```python
from build123d import *

# Parameters (mm, degrees)
SKETCH_1_R          = 1.6
SKETCH_1_W          = 15.2
SKETCH_1_H          = 15.2
EXTRUDE_1_DEPTH     = 19.5
CUT_EXTRUDE_1_DEPTH = 14.5
SKETCH_3_W          = 23.2
SKETCH_3_H          = 23.2
SKETCH_3_W_2        = 15.2
SKETCH_3_H_2        = 15.2
EXTRUDE_2_DEPTH     = 20
FILLET_1_R          = 4
FILLET_2_R          = 6
CHAMFER_1_SIZE      = 1.5
CHAMFER_2_SIZE      = 1
SKETCH_4_R          = 1.6
CUT_EXTRUDE_2_DEPTH = 68.026114314
SKETCH_5_R          = 1.6
CUT_EXTRUDE_3_DEPTH = 68.026114314
FILLET_3_R          = 5


with BuildPart() as part:
    # 草图1 → 凸台-拉伸1 (new body)
    with BuildSketch(Plane(origin=(0, 0, 0), x_dir=(0, 0, -1), z_dir=(1, 0, 0))):
        Polygon((12.5, -30.7), (30.7, -30.7), (30.7, -12.5), (40, -12.5), (40, 12.5), (-12.5, 12.5), (-12.5, -40), (12.5, -40), align=None)
        with Locations((10, 0)):
            Circle(SKETCH_1_R, mode=Mode.SUBTRACT)
        with Locations((30, 0)):
            Circle(SKETCH_1_R, mode=Mode.SUBTRACT)
        with Locations(Location((0, -30, 0), (0, 0, 180))):
            Circle(SKETCH_1_R, mode=Mode.SUBTRACT)
        with Locations(Location((0, -10, 0), (0, 0, 180))):
            Circle(SKETCH_1_R, mode=Mode.SUBTRACT)
        with Locations((15.1, -15.1)):
            Rectangle(SKETCH_1_W, SKETCH_1_H, mode=Mode.SUBTRACT)
    extrude(amount=EXTRUDE_1_DEPTH)

    # 草图2 → 切除-拉伸1 (cut)
    with BuildSketch(Plane.ZY):
        Polygon((7.5, 7.5), (7.5, -40), (-7.5, -40), (-7.5, -7.5), (-40, -7.5), (-40, 7.5), align=None)
    extrude(amount=-CUT_EXTRUDE_1_DEPTH, mode=Mode.SUBTRACT)

    # 草图3 → 凸台-拉伸2 (add)
    with BuildSketch(Plane(origin=(19.5, 0, 0), x_dir=(0, 0, -1), z_dir=(1, 0, 0))):
        with Locations((15.1, -15.1)):
            Rectangle(SKETCH_3_W, SKETCH_3_H)
        with Locations((15.1, -15.1)):
            Rectangle(SKETCH_3_W_2, SKETCH_3_H_2, mode=Mode.SUBTRACT)
    extrude(amount=EXTRUDE_2_DEPTH)

    # 圆角1
    # the kernel refuses this fillet: 4 mm, written as the material it adds along each edge
    with BuildSketch(Plane(origin=(19.5, -3.5, -3.5), x_dir=(0, 0, 1), z_dir=(0, -1, 0))) as fillet_1_piece_1_section:
        with BuildLine():
            CenterArc((FILLET_1_R, -FILLET_1_R), FILLET_1_R, 90, 90)
            Line((0, -FILLET_1_R), (0, 0))
            Line((0, 0), (FILLET_1_R, 0))
        make_face()
    fillet_1_piece_1 = extrude(amount=23.2, mode=Mode.PRIVATE)
    fillet_1_piece_1 = fillet_1_piece_1 - Plane(origin=(20.41689995, -10, 0), x_dir=(0, 0, 1), z_dir=(-1, 0, 0)) * Cylinder(1.6, 63, mode=Mode.PRIVATE)
    add(fillet_1_piece_1)
    with BuildSketch(Plane(origin=(19.5, -26.7, -3.5), x_dir=(0, -1, 0), z_dir=(0, 0, -1)), Plane(origin=(19.5, -26.7, -26.7), x_dir=(0, 0, -1), z_dir=(0, 1, 0))) as fillet_1_piece_2:
        with BuildLine():
            CenterArc((FILLET_1_R, -FILLET_1_R), FILLET_1_R, 90, 90)
            Line((0, -FILLET_1_R), (0, 0))
            Line((0, 0), (FILLET_1_R, 0))
        make_face()
    extrude(amount=23.2)
    with BuildSketch(Plane(origin=(19.5, -3.5, -26.7), x_dir=(0, 1, 0), z_dir=(0, 0, 1))) as fillet_1_piece_3_section:
        with BuildLine():
            CenterArc((FILLET_1_R, -FILLET_1_R), FILLET_1_R, 90, 90)
            Line((0, -FILLET_1_R), (0, 0))
            Line((0, 0), (FILLET_1_R, 0))
        make_face()
    fillet_1_piece_3 = extrude(amount=23.2, mode=Mode.PRIVATE)
    fillet_1_piece_3 = fillet_1_piece_3 - Plane(origin=(20.416900014, 0, -10), x_dir=(0, 0, -1), z_dir=(-1, 0, 0)) * Cylinder(1.6, 63, mode=Mode.PRIVATE)
    add(fillet_1_piece_3)
    with BuildSketch(Plane(origin=(19.5, -3.5, -26.7), x_dir=(0, 1, 0), z_dir=(0, 0, 1))) as fillet_1_piece_4a_section:
        with BuildLine():
            CenterArc((FILLET_1_R, -FILLET_1_R), FILLET_1_R, 90, 90)
            Line((0, -FILLET_1_R), (0, 0))
            Line((0, 0), (FILLET_1_R, 0))
        make_face()
    fillet_1_piece_4a = extrude(amount=33.2, mode=Mode.PRIVATE)
    fillet_1_piece_4a = split(fillet_1_piece_4a, bisect_by=Plane(origin=(20.405580457, -2.594419543, -3.5), z_dir=(0, 0, 1)), keep=Keep.TOP, mode=Mode.PRIVATE)
    with BuildSketch(Plane(origin=(19.5, 6.5, -3.5), x_dir=(0, 0, 1), z_dir=(0, -1, 0))) as fillet_1_piece_4b_section:
        with BuildLine():
            CenterArc((FILLET_1_R, -FILLET_1_R), FILLET_1_R, 90, 90)
            Line((0, -FILLET_1_R), (0, 0))
            Line((0, 0), (FILLET_1_R, 0))
        make_face()
    fillet_1_piece_4b = extrude(amount=33.2, mode=Mode.PRIVATE)
    fillet_1_piece_4b = split(fillet_1_piece_4b, bisect_by=Plane(origin=(20.405580457, -3.5, -2.594419543), z_dir=(0, 1, 0)), keep=Keep.TOP, mode=Mode.PRIVATE)
    fillet_1_piece_4 = fillet_1_piece_4a & fillet_1_piece_4b
    add(fillet_1_piece_4)
    with BuildSketch(Plane(origin=(19.5, -26.7, 6.5), x_dir=(0, -1, 0), z_dir=(0, 0, -1))) as fillet_1_piece_5a_section:
        with BuildLine():
            CenterArc((FILLET_1_R, -FILLET_1_R), FILLET_1_R, 90, 90)
            Line((0, -FILLET_1_R), (0, 0))
            Line((0, 0), (FILLET_1_R, 0))
        make_face()
    fillet_1_piece_5a = extrude(amount=33.2, mode=Mode.PRIVATE)
    fillet_1_piece_5a = fillet_1_piece_5a - Plane(origin=(20.438690709, -30, 0), x_dir=(0, 0, 1), z_dir=(-1, 0, 0)) * Cylinder(1.6, 83, mode=Mode.PRIVATE)
    fillet_1_piece_5a = split(fillet_1_piece_5a, bisect_by=Plane(origin=(20.438690709, -27.535460333, -3.5), z_dir=(0, 0, 1)), keep=Keep.TOP, mode=Mode.PRIVATE)
    with BuildSketch(Plane(origin=(19.5, -3.5, -3.5), x_dir=(0, 0, 1), z_dir=(0, -1, 0))) as fillet_1_piece_5b_section:
        with BuildLine():
            CenterArc((FILLET_1_R, -FILLET_1_R), FILLET_1_R, 90, 90)
            Line((0, -FILLET_1_R), (0, 0))
            Line((0, 0), (FILLET_1_R, 0))
        make_face()
    fillet_1_piece_5b = extrude(amount=33.2, mode=Mode.PRIVATE)
    fillet_1_piece_5b = fillet_1_piece_5b - Plane(origin=(20.432327139, -30, 0), x_dir=(0, 0, 1), z_dir=(-1, 0, 0)) * Cylinder(1.6, 83, mode=Mode.PRIVATE)
    fillet_1_piece_5b = split(fillet_1_piece_5b, bisect_by=Plane(origin=(20.432327139, -26.7, -2.653974982), z_dir=(0, -1, 0)), keep=Keep.TOP, mode=Mode.PRIVATE)
    fillet_1_piece_5 = fillet_1_piece_5a & fillet_1_piece_5b
    add(fillet_1_piece_5)
    with BuildSketch(Plane(origin=(19.5, -26.7, -3.5), x_dir=(0, -1, 0), z_dir=(0, 0, -1))) as fillet_1_piece_6a_section:
        with BuildLine():
            CenterArc((FILLET_1_R, -FILLET_1_R), FILLET_1_R, 90, 90)
            Line((0, -FILLET_1_R), (0, 0))
            Line((0, 0), (FILLET_1_R, 0))
        make_face()
    fillet_1_piece_6a = extrude(amount=33.2, mode=Mode.PRIVATE)
    fillet_1_piece_6a = split(fillet_1_piece_6a, bisect_by=Plane(origin=(20.405580457, -27.605580457, -30.7), z_dir=(0, 0, 1)), keep=Keep.TOP, mode=Mode.PRIVATE)
    fillet_1_piece_6a = split(fillet_1_piece_6a, bisect_by=Plane(origin=(20.405580457, -27.605580457, -26.7), z_dir=(0, 0, -1)), keep=Keep.TOP, mode=Mode.PRIVATE)
    with BuildSketch(Plane(origin=(19.5, -36.7, -26.7), x_dir=(0, 0, -1), z_dir=(0, 1, 0))) as fillet_1_piece_6b_section:
        with BuildLine():
            CenterArc((FILLET_1_R, -FILLET_1_R), FILLET_1_R, 90, 90)
            Line((0, -FILLET_1_R), (0, 0))
            Line((0, 0), (FILLET_1_R, 0))
        make_face()
    fillet_1_piece_6b = extrude(amount=33.2, mode=Mode.PRIVATE)
    fillet_1_piece_6b = split(fillet_1_piece_6b, bisect_by=Plane(origin=(20.405580457, -30.7, -27.605580457), z_dir=(0, 1, 0)), keep=Keep.TOP, mode=Mode.PRIVATE)
    fillet_1_piece_6b = split(fillet_1_piece_6b, bisect_by=Plane(origin=(20.405580457, -26.7, -27.605580457), z_dir=(0, -1, 0)), keep=Keep.TOP, mode=Mode.PRIVATE)
    fillet_1_piece_6 = fillet_1_piece_6a & fillet_1_piece_6b
    add(fillet_1_piece_6)
    with BuildSketch(Plane(origin=(19.5, -26.7, -26.7), x_dir=(0, 0, -1), z_dir=(0, 1, 0))) as fillet_1_piece_7a_section:
        with BuildLine():
            CenterArc((FILLET_1_R, -FILLET_1_R), FILLET_1_R, 90, 90)
            Line((0, -FILLET_1_R), (0, 0))
            Line((0, 0), (FILLET_1_R, 0))
        make_face()
    fillet_1_piece_7a = extrude(amount=33.2, mode=Mode.PRIVATE)
    fillet_1_piece_7a = fillet_1_piece_7a - Plane(origin=(20.438690575, 0, -30), x_dir=(0, 0, -1), z_dir=(-1, 0, 0)) * Cylinder(1.6, 83, mode=Mode.PRIVATE)
    fillet_1_piece_7a = split(fillet_1_piece_7a, bisect_by=Plane(origin=(20.438690575, -3.5, -27.535460712), z_dir=(0, 1, 0)), keep=Keep.TOP, mode=Mode.PRIVATE)
    with BuildSketch(Plane(origin=(19.5, -3.5, -36.7), x_dir=(0, 1, 0), z_dir=(0, 0, 1))) as fillet_1_piece_7b_section:
        with BuildLine():
            CenterArc((FILLET_1_R, -FILLET_1_R), FILLET_1_R, 90, 90)
            Line((0, -FILLET_1_R), (0, 0))
            Line((0, 0), (FILLET_1_R, 0))
        make_face()
    fillet_1_piece_7b = extrude(amount=33.2, mode=Mode.PRIVATE)
    fillet_1_piece_7b = fillet_1_piece_7b - Plane(origin=(20.432327238, 0, -30), x_dir=(0, 0, -1), z_dir=(-1, 0, 0)) * Cylinder(1.6, 83, mode=Mode.PRIVATE)
    fillet_1_piece_7b = split(fillet_1_piece_7b, bisect_by=Plane(origin=(20.432327238, -2.653975394, -26.7), z_dir=(0, 0, -1)), keep=Keep.TOP, mode=Mode.PRIVATE)
    fillet_1_piece_7 = fillet_1_piece_7a & fillet_1_piece_7b
    add(fillet_1_piece_7)

    # 圆角2
    # the kernel refuses this fillet: 6 mm, written as the material it adds along each edge
    with BuildSketch(Plane(origin=(0, -30.7, -12.5), x_dir=(0, 0, -1), z_dir=(1, 0, 0)), Plane(origin=(0, -12.5, -30.7), x_dir=(0, 0, -1), z_dir=(1, 0, 0))) as fillet_2_piece_1:
        with BuildLine():
            CenterArc((FILLET_2_R, -FILLET_2_R), FILLET_2_R, 90, 90)
            Line((0, -FILLET_2_R), (0, 0))
            Line((0, 0), (FILLET_2_R, 0))
        make_face()
    extrude(amount=19.5)
    # the kernel refuses this fillet: 6 mm, written as the material it takes off along each edge
    with BuildSketch(Plane(origin=(-15, -30.7, -30.7), x_dir=(0, 0, 1), z_dir=(1, 0, 0))) as fillet_2_2_piece_1:
        with BuildLine():
            CenterArc((FILLET_2_R, -FILLET_2_R), FILLET_2_R, 90, 90)
            Line((0, -FILLET_2_R), (0, 0))
            Line((0, 0), (FILLET_2_R, 0))
        make_face()
    extrude(amount=49.5, mode=Mode.SUBTRACT)

    # 倒角1
    chamfer_1_edges = [part.edges().sort_by_distance(p)[0] for p in [
        (39.5, -15.1, -7.5),
        (39.5, -22.7, -15.1),
        (39.5, -15.1, -22.7),
        (39.5, -7.5, -15.1),
    ]]
    chamfer(chamfer_1_edges, length=CHAMFER_1_SIZE)

    # 倒角2
    chamfer_2_edges = [part.edges().sort_by_distance(p)[0] for p in [
        (0, 7.5, -16.25),
        (0, -7.5, -31.35),
        (0, -31.35, -7.5),
        (0, -16.25, 7.5),
    ]]
    chamfer(chamfer_2_edges, length=CHAMFER_2_SIZE)

    # 草图4 → 切除-拉伸2 (cut, through all)
    with BuildSketch(Plane.XY.offset(-3.5)):
        with Locations((32, -15.1)):
            Circle(SKETCH_4_R)
    extrude(amount=-CUT_EXTRUDE_2_DEPTH, mode=Mode.SUBTRACT)

    # 草图5 → 切除-拉伸3 (cut, through all)
    with BuildSketch(Plane(origin=(0, -3.5, 0), x_dir=(1, 0, 0), z_dir=(0, 1, 0))):
        with Locations(Location((32, 15.1, 0), (0, 0, 270))):
            Circle(SKETCH_5_R)
    extrude(amount=-CUT_EXTRUDE_3_DEPTH, mode=Mode.SUBTRACT)

    # 圆角3
    fillet_3_edges = [part.edges().sort_by_distance(p)[0] for p in [
        (9.75, 12.5, 12.5),
    ]]
    fillet(fillet_3_edges, radius=FILLET_3_R)


solid = part.part
```
Geometry check sheet. Reference: the model listing, model coordinates, mm. A direction names the side the tool comes from. Coordinates: 2 decimals unless noted, no trailing zeros. Write each loop counter-clockwise with the first axis right and the second up, starting at its lowest first coordinate (ties: lowest second). Pieces come first, ordered by that corner, then holes. Notation, with made-up numbers: (12, 25) -> (70, 25) arc R18 cw to (70, 46) -> close; hole circle Ø5 at (68, 33). An arc over 180 degrees is marked (long way). Use CSV: the item, a comma, the result in double quotes. Start each with the question number.
Item 1: Cross-section at B-B, the plane y = -10. Record the cut outline in (x, z).
Item 2: Mould release check, pull along X, two halves, no side actions. Record for faces 4 (the flat face through (30, -3.5, -15)), 5 (the cylindrical face through (31.39, -24.67, -13.62)), 6 (the flat face through (14.5, -5, -11)), 7 (the cylindrical face through (20.641, -27.903, -14.891)): released by +X, released by -X, zero draft, split by the parting line, or undercut.
Item 3: Cross-section at A-A, the plane x = 32. Record the cut outline in (y, z), plus the area to 3 significant figures.
Item 4: Cross-section at D-D, the plane x = 7. Record the cut outline in (y, z), plus the area to 3 significant figures.
Item 5: Set-up check for faces 1 (the flat face through (8, 7.5, -17)), 2 (the flat face through (38.8, -15.2, -23.5)), 3 (the flat face through (10, -30.7, -22)): record each of +Z, -Z, +X, -X, +Y, -Y from which the full face is reachable in a straight line by a thin tool's end or side.
Item 6: Depth check by flat-ended pin: pin 1 Ø17.5 at (x, z) = (32.5, -17.5) entering from +Y; pin 2 Ø2 at (x, z) = (32, -27) entering from -Y; pin 3 Ø3 at (y, z) = (2, -10.5) entering from -X; pin 4 Ø2.5 at (x, y) = (32, -15.1) entering from -Z. Enter the tip coordinate at first touch or a pass-through.
Item 7: Thickness scan on line 1 (Z direction, x = 15, y = -10); line 2 (Y direction, x = 15, z = 0). Record the ranges inside material, lowest first.
Answers:
1,outline,"(0, -40) -> (19.5, -40) -> (19.5, -30.7) arc R4 cw to (23.5, -26.7) -> (39.5, -26.7) -> (39.5, -24.2) -> (38, -22.7) -> (0, -22.7) -> close; (0, 8.5) -> (1, 7.5) -> (14.5, 7.5) -> (14.5, 1.6) -> (19.5, 1.6) -> (19.5, 12.5) -> (0, 12.5) -> close; (14.5, -7.5) -> (38, -7.5) -> (39.5, -6) -> (39.5, -3.5) -> (23.5, -3.5) arc R4 cw to (20.1, -1.6) -> (14.5, -1.6) -> close"
2,face 4,"zero draft"
2,face 5,"undercut"
2,face 6,"released by -X"
2,face 7,"released by +X"
3,outline,"(-26.7, -26.7) -> (-16.7, -26.7) -> (-16.7, -22.7) -> (-22.7, -22.7) -> (-22.7, -16.7) -> (-26.7, -16.7) -> close; (-26.7, -13.5) -> (-22.7, -13.5) -> (-22.7, -7.5) -> (-16.7, -7.5) -> (-16.7, -3.5) -> (-26.7, -3.5) -> close; (-13.5, -26.7) -> (-3.5, -26.7) -> (-3.5, -16.7) -> (-7.5, -16.7) -> (-7.5, -22.7) -> (-13.5, -22.7) -> close; (-13.5, -7.5) -> (-7.5, -7.5) -> (-7.5, -13.5) -> (-3.5, -13.5) -> (-3.5, -3.5) -> (-13.5, -3.5) -> close"
3,area,"256 mm^2"
4,outline,"(-40, -12.5) -> (-36.7, -12.5) arc R6 cw to (-30.7, -18.5) -> (-30.7, -24.7) arc R6 ccw to (-24.7, -30.7) -> (-18.5, -30.7) arc R6 cw to (-12.5, -36.7) -> (-12.5, -40) -> (-7.5, -40) -> (-7.5, -22.7) -> (-22.7, -22.7) -> (-22.7, -7.5) -> (-40, -7.5) -> close; (-40, 7.5) -> (7.5, 7.5) -> (7.5, -40) -> (12.5, -40) -> (12.5, 7.5) arc R5 ccw to (7.5, 12.5) -> (-40, 12.5) -> close"
4,area,"903 mm^2"
5,face 1,"-Z, -X"
5,face 2,"+X"
5,face 3,"-Z, +X, -X, -Y"
6,pin 1,"y = -3.5"
6,pin 2,"y = -26.7"
6,pin 3,"x = 14.5"
6,pin 4,"through"
7,line 1,"-40 to -22.7, -7.5 to -1.6, 1.6 to 12.5"
7,line 2,"-40 to -31.6, -28.4 to -11.6, -8.4 to 12.5"
